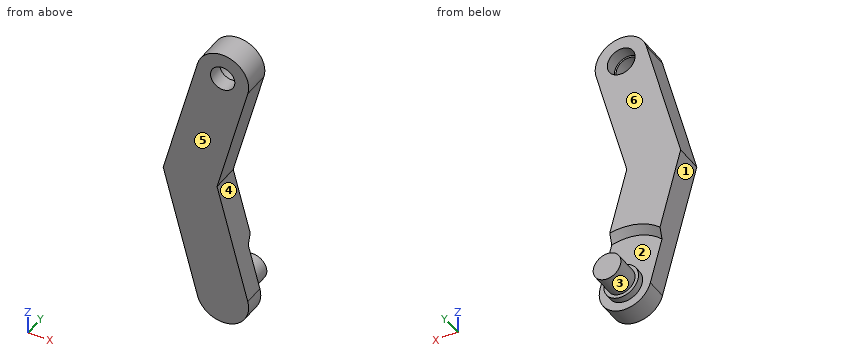
Autodesk Inventor part; units mm, degrees
ref_plane "YZ Plane" through (0, 0, 0) normal (1, 0, 0) x (0, 1, 0)
ref_plane "XZ Plane" through (0, 0, 0) normal (0, 1, 0) x (-1, 0, 0)
ref_plane "XY Plane" through (0, 0, 0) normal (0, 0, 1) x (1, 0, 0)
sketch "Sketch3" plane through (0, 0, 0) normal (0, 1, 0) x (-1, 0, 0)
  circle A0 centre (0, 0) radius 4
  circle A1 centre (0, 0) radius 5
  circle A2 centre (0, 0) radius 7.5
  line L0 (0, -24.5) -> (0, 94.5)
  line L1 (22.0714, 0) -> (-12.4286, 0)
  circle A3 centre (0, 70) radius 4
  line L2 (7.2444, -1.9411) -> (17.1428, 35)
  line L3 (17.1428, 35) -> (7.2444, 71.9411)
  circle A4 centre (0, 70) radius 7.5
  line L4 (-7.2444, 1.9411) -> (1.6137, 35)
  line L5 (1.6137, 35) -> (-7.2444, 68.0589)
  circle A5 centre (0, 70) radius 3.5
  dimension "d15" = 8
  dimension "d16" = 10
  dimension "d17" = 15
  dimension "d18" = 8
  dimension "d19" = 70
  dimension "d20" = 15
  dimension "d21" = 35
  dimension "d24" = 15
  dimension "d25" = 35
  dimension "d43" = 7
extrude "Extrusion4" add sketch "Sketch3" along normal blind 8 contours L1 L2 A2 | A2 L0 L4 L5 A4 L3 L2 L1 | A2 L4 L0 | L5 A4 L0
extrude "Extrusion5" add sketch "Sketch3" along normal blind 8 contours L1 A2 L0 A1 | A1 L0 A2 L1 | A1 L1 A2 L0 | L0 A2 L1 A1
sketch "Sketch4" plane through (0, 8, 0) normal (0, 1, 0) x (1, 0, 0)
  circle A0 centre (0, 0) radius 15
  circle A1 centre (0, 0) radius 13.25
  dimension "d30" = 30
  dimension "d31" = 26.5
extrude "Extrusion6" cut sketch "Sketch4" against normal blind 2 contours A0 | A1
extrude "Extrusion7" add sketch "Sketch3" along normal blind 15 contours L1 L0 A0 | A0 L0 L1 | L0 L1 A0 | A0 L1 L0
extrude "Extrusion8" add sketch "Sketch3" along normal blind 8 contours L1 A1 L0 A0 | A0 L0 A1 L1 | A0 L1 A1 L0 | L0 A1 L1 A0
chamfer "Chamfer1" distance 2 angle 45 1 edges at (-3.8823, 8, 14.4889)
extrude "Extrusion9" add sketch "Sketch3" along normal blind 8 contours A4 L0 A3 | A4 L0 A3
extrude "Extrusion10" add sketch "Sketch3" along normal blind 4.5 contours A3 L0 A5 | L0 A5 A3
properties part number "side arm"
For this review, take the finished solid that the model builds, in its own axes (mm). Face numbers are marked on the shaded views. A direction names the side the tool comes from. Round coordinates to 2 decimals unless told otherwise and drop trailing zeros. Order: outer loops, then holes, each group sorted by start corner. A loop starts at its lowest first (then second) coordinate and runs counter-clockwise, first axis right, second up. Notation, with made-up numbers: M 38,78.5 L 50,78.5 A17 cw 50,99.5 Z; hole C -33.5,32 d9. An arc over 180 degrees is marked long. Write each question's results on one line, items separated by ' | '. Start each with the question number.
1. Draft analysis for pull direction Z (two halves, no side actions). For the marked faces 1, 2, 3 and 4, state which applies: pulls with the +Z half, pulls with the -Z half, needs draft (parallel to the pull), parting line crosses it, or undercut.
2. Add section C-C (x = 0). State how many separate pieces and enclosed holes the cut face has, then the cut area to 3 significant figures.
3. Tool access review of the marked faces 5 and 6: name each direction out of +Z, -Z, +X, -X, +Y, -Y from which nothing blocks a thin tool from reaching the whole face with its end or side.
4. To check wall thickness, follow L1, parallel to Y at x = -5, z = 32.5; L2, parallel to Z at x = -3, y = 6.75; L3, parallel to X at y = 5.6, z = 70. State the ranges of each line that lie inside material, in increasing order. Write a range as [from, to].
5. Add section A-A (z = 70). State the section outline as (x, y) points.
6. Clearance check with flat-ended pins moving along their axes: pin 1 Ø6 at (y, z) = (7, 24) entering from -X; pin 2 Ø12 at (x, z) = (-9.5, 20) entering from +Y; pin 3 Ø2 at (y, z) = (4.5, 56) entering from -X. State where each tip first meets the part, or that it passes through.
7. Add section D-D (y = 14.25). State the section outline as (x, z) points.
Output values:
1) face 1: pulls with the -Z half | face 2: undercut | face 3: parting line crosses it | face 4: undercut
2) separate pieces: 3 | enclosed holes: 0 | area: 553 mm^2
3) face 5: +Z, -Z, +X, -X, -Y | face 6: +Z, +X, -X, +Y
4) L1: [0, 8] | L2: [-4, 4], [15.46, 67.35], [72.65, 76.87] | L3: [-7.76, -4], [4, 7.5]
5) outline: M -7.76,0 L -3.5,0 L -3.5,4.5 L -4,4.5 L -4,8 L -7.76,8 Z; M 3.5,0 L 7.5,0 L 7.5,8 L 4,8 L 4,4.5 L 3.5,4.5 Z
6) pin 1: x = -15 | pin 2: y = 8 | pin 3: x = -11.78
7) outline: C 0,0 d8
